Here's how the part is built. I have some questions about the finished solid (model axes, mm). A direction names the side the tool comes from. Give positions to 0.01 mm unless a question says otherwise; leave off trailing zeros. Write each loop counter-clockwise with the first axis right and the second up, starting at its lowest first coordinate (ties: lowest second). Pieces come first, ordered by that corner, then holes. Notation, with made-up numbers: (10.25, -2) -> (31.25, -2) arc R34 ccw to (31.25, 36) -> close; hole circle Ø3 at (-39.5, -15). An arc over 180 degrees is marked (long way). Use one line per item in the form item = value.
```python
from build123d import *

# Parameters (mm, degrees)
SKETCH1_R               = 1
SKETCH1_W               = 3.1
SKETCH1_H               = 3.1
BOSS_EXTRUDE1_DEPTH     = 2
BOSS_EXTRUDE2_DEPTH     = 3
SKETCH4_W               = 3.1
SKETCH4_H               = 3.1
BOSS_EXTRUDE3_DEPTH     = 0.5
SKETCH5_W               = 3.7
SKETCH5_H               = 3.7
CUT_EXTRUDE1_DEPTH      = 1.5
CUT_EXTRUDE2_DEPTH      = 64.401025228
CUT_EXTRUDE2_DEPTH_BACK = 64.401025228
SKETCH6_R               = 1.5


with BuildPart() as part:
    # Sketch1 → Boss-Extrude1 (new body)
    with BuildSketch(Plane(origin=(0, 0, 0), x_dir=(1, 0, 0), z_dir=(0, 1, 0))):
        Polygon((-5, 52.5), (-5, 22.5), (5, 22.5), (5, 52.5), (35, 52.5), (35, -52.5), (-35, -52.5), (-35, 52.5), align=None)
        with Locations(Location((-9.049911388, 48.178259549, 0), (0, 0, 270))):
            Circle(SKETCH1_R, mode=Mode.SUBTRACT)
        with Locations(Location((-9.049911388, 30.178259549, 0), (0, 0, 270))):
            Circle(SKETCH1_R, mode=Mode.SUBTRACT)
        with Locations((-30, -32.05)):
            Rectangle(SKETCH1_W, SKETCH1_H, mode=Mode.SUBTRACT)
        with Locations((30, -32.05)):
            Rectangle(SKETCH1_W, SKETCH1_H, mode=Mode.SUBTRACT)
    extrude(amount=BOSS_EXTRUDE1_DEPTH)

    # Sketch3 → Boss-Extrude2 (add)
    with BuildSketch(Plane(origin=(35, 0, 0), x_dir=(0, 0, -1), z_dir=(1, 0, 0))):
        with BuildLine():
            Line((-33.25, 0), (-35.25, 0))
            Line((-35.25, 0), (-35.25, -1.1))
            ThreePointArc((-35.25, -1.1), (-32.15, -4.2), (-29.05, -1.1))
            Line((-29.05, -1.1), (-29.05, 0))
            Line((-29.05, 0), (-31.05, 0))
            Line((-31.05, 0), (-31.05, -1.1))
            ThreePointArc((-31.05, -1.1), (-32.15, -2.2), (-33.25, -1.1))
            Line((-33.25, -1.1), (-33.25, 0))
        make_face()
    boss_extrude2 = extrude(amount=-BOSS_EXTRUDE2_DEPTH)

    # Mirror1: Boss-Extrude2 across plane
    add(boss_extrude2.mirror(Plane(origin=(0, 0, 0), x_dir=(0, 0, 1), z_dir=(1, 0, 0))))

    # Sketch4 → Boss-Extrude3 (add)
    with BuildSketch(Plane.XZ):
        with Locations((-30, 32.05)):
            Rectangle(SKETCH4_W, SKETCH4_H)
        with Locations((30, 32.05)):
            Rectangle(SKETCH4_W, SKETCH4_H)
    extrude(amount=-BOSS_EXTRUDE3_DEPTH)

    # Sketch5 → Cut-Extrude1 (cut)
    with BuildSketch(Plane(origin=(0, 2, 0), x_dir=(1, 0, 0), z_dir=(0, 1, 0))):
        with Locations((-30, -32.05)):
            Rectangle(SKETCH5_W, SKETCH5_H)
        with Locations((30, -32.05)):
            Rectangle(SKETCH5_W, SKETCH5_H)
    extrude(amount=-CUT_EXTRUDE1_DEPTH, mode=Mode.SUBTRACT)

    # Sketch6 → Cut-Extrude2 (cut, two sides: drawn at the far end of the back side and taken through both)
    with BuildSketch(Plane(origin=(0, 2, 0), x_dir=(1, 0, 0), z_dir=(0, 1, 0)).offset(-CUT_EXTRUDE2_DEPTH_BACK)):
        with Locations(Location((-8.95, 19.5, 0), (0, 0, 270))):
            Circle(SKETCH6_R)
        with Locations(Location((18.95, 19.5, 0), (0, 0, 270))):
            Circle(SKETCH6_R)
        with Locations(Location((24.05, -32.6, 0), (0, 0, 270))):
            Circle(SKETCH6_R)
        with Locations(Location((-24.15, -31.3, 0), (0, 0, 270))):
            Circle(SKETCH6_R)
    extrude(amount=CUT_EXTRUDE2_DEPTH + CUT_EXTRUDE2_DEPTH_BACK, mode=Mode.SUBTRACT)


solid = part.part
```
Q1. I want a section at C-C, the plane x = 30. Write out the boundary of the cut face in (y, z).
Result set:
outline = (0, -52.5) -> (2, -52.5) -> (2, 30.2) -> (0.5, 30.2) -> (0.5, 33.9) -> (2, 33.9) -> (2, 52.5) -> (0, 52.5) -> close
Q2. Will these pins go through, and if not, where does the flat tip stop? pin 1 Ø0.9 at (x, y) = (34, -0.5) entering from +Z; pin 2 Ø0.9 at (x, y) = (-33, -0.5) entering from -Z; pin 3 Ø3.5 at (y, z) = (-1.5, 32.5) entering from +X; pin 4 Ø1 at (x, z) = (24.5, -17) entering from -Y.
Result set:
pin_1 = 35.25
pin_2 = 29.05
pin_3 = 35
pin_4 = 0
Q3. If I drill on line 1 along X through (y, z) = (1.3, -19.5); line 2 along Z through (x, y) = (-8.95, 0.8); line 3 along Z through (x, y) = (24, 0.75), over which ranges is the centre line in solid material (lowest first)? Write a range as from..to.
Result set:
line_1 = -35..-10.45, -7.45..17.45, 20.45..35
line_2 = -52.5..-49.17, -47.18..-31.17, -29.18..-21, -18..52.5
line_3 = -52.5..31.1, 34.1..52.5
Q4. Which directions (+Z, -Z, +X, -X, +Y, -Y) give clear straight access to the entire face, cutting with the end or side of a thin tool? Please do faces 1 (the face through (-30, 0.5, 32)), 2 (the face through (-5, 1, -38)), 3 (the face through (0, 2, -1)).
Result set:
face_1 = +Y
face_2 = -Z, +Y, -Y
face_3 = +Z, -Z, +X, -X, +Y
Q5. I want a section at D-D, the plane z = 37. Write out the boundary of the cut face in (x, y), and give its area (3 significant figures).
Result set:
outline = (-35, 0) -> (35, 0) -> (35, 2) -> (-35, 2) -> close
area = 140 mm2
Q6. I want a section at B-B, the plane z = -45.5. Write out the boundary of the cut face in (x, y), and give its area (3 significant figures).
Result set:
outline = (-35, 0) -> (-5, 0) -> (-5, 2) -> (-35, 2) -> close; (5, 0) -> (35, 0) -> (35, 2) -> (5, 2) -> close
area = 120 mm2
Q7. I want a section at A-A, the plane x = 18.95. Write out the boundary of the cut face in (y, z), and give its area (3 significant figures).
Result set:
outline = (0, -52.5) -> (2, -52.5) -> (2, -21) -> (0, -21) -> close; (0, -18) -> (2, -18) -> (2, 52.5) -> (0, 52.5) -> close
area = 204 mm2
Q8. If we mould it in two halves opening along Y, with no side actions, what happens to faces 4 (the face through (33.5, -2.2, 32.1)), 5 (the face through (35, 0.2, -0.7)), 6 (the face through (-33.5, -4.2, 32.2))? For each: +Y half, -Y half, draft (parallel to the pull), parting line (faces both ways), or undercut.
Result set:
face_4 = undercut
face_5 = draft
face_6 = -Y half
